Build history of the part. All positions in model axes, mm. Face numbers are marked on the shaded views. A direction names the side the tool comes from. Round coordinates to 2 decimals unless told otherwise and drop trailing zeros. Order: outer loops, then holes, each group sorted by start corner. A loop starts at its lowest first (then second) coordinate and runs counter-clockwise, first axis right, second up. Notation, with made-up numbers: M 30,34 L 35,34 A11 cw 35,51 Z; hole C -30,79.5 d4. An arc over 180 degrees is marked long. Use CSV: the item, a comma, the result in double quotes.
from build123d import *

# Parameters (mm, degrees)
SKETCH_1_W          = 26
SKETCH_1_H          = 25
EXTRUDE_1_DEPTH     = 20
EXTRUDE_3_DEPTH     = 26
SKETCH_4_W          = 26
SKETCH_4_H          = 18
EXTRUDE_4_DEPTH     = 10
SKETCH_5_W          = 22.5
SKETCH_5_H          = 12.5
CUT_EXTRUDE_1_DEPTH = 23.05
CUT_EXTRUDE_5_DEPTH = 3.55
SKETCH_9_W          = 7
SKETCH_9_H          = 8
CUT_EXTRUDE_6_DEPTH = 2
SKETCH_10_W         = 2
SKETCH_10_H         = 8
CUT_EXTRUDE_7_DEPTH = 2
EXTRUDE_5_DEPTH     = 26
FILLET_1_R          = 2


with BuildPart() as part:
    # Эскиз1 → Бобышка-Вытянуть1 (new body)
    with BuildSketch(Plane.XY):
        Rectangle(SKETCH_1_W, SKETCH_1_H)
    extrude(amount=EXTRUDE_1_DEPTH)

    # Эскиз3 → Бобышка-Вытянуть3 (add, through all)
    with BuildSketch(Plane(origin=(13, 0, 0), x_dir=(0, 0, -1), z_dir=(1, 0, 0))):
        with BuildLine():
            Line((-20, 12.5), (-21.75, 12.5))
            ThreePointArc((-21.75, 12.5), (-23, 11.25), (-21.75, 10))
            Line((-21.75, 10), (-20, 10))
            Line((-20, 10), (-20, 12.5))
        make_face()
    extrude_3 = extrude(amount=-EXTRUDE_3_DEPTH)

    # Зеркальное отражение1: Бобышка-Вытянуть3 across plane
    add(extrude_3.mirror(Plane.ZX))

    # Эскиз4 → Бобышка-Вытянуть4 (add)
    with BuildSketch(Plane.XY.offset(20)):
        Rectangle(SKETCH_4_W, SKETCH_4_H)
    extrude(amount=EXTRUDE_4_DEPTH)

    # Эскиз5 → Вырез-Вытянуть1 (cut)
    with BuildSketch(Plane.XY.offset(30)):
        Rectangle(SKETCH_5_W, SKETCH_5_H)
    extrude(amount=-CUT_EXTRUDE_1_DEPTH, mode=Mode.SUBTRACT)

    # Эскиз8 → Вырез-Вытянуть5 (cut)
    with BuildSketch(Plane.ZY.offset(13)):
        with BuildLine():
            Line((30, -6.25), (13.2, -6.25))
            ThreePointArc((13.2, -6.25), (6.95, 0), (13.2, 6.25))
            Line((13.2, 6.25), (30, 6.25))
            Line((30, 6.25), (30, -6.25))
        make_face()
    extrude(amount=-CUT_EXTRUDE_5_DEPTH, mode=Mode.SUBTRACT)

    # Эскиз9 → Вырез-Вытянуть6 (cut)
    with BuildSketch(Plane.XY.offset(6.95)):
        with Locations((7.7560221, 0)):
            Rectangle(SKETCH_9_W, SKETCH_9_H)
    extrude(amount=-CUT_EXTRUDE_6_DEPTH, mode=Mode.SUBTRACT)

    # Эскиз10 → Вырез-Вытянуть7 (cut)
    with BuildSketch(Plane.ZY.offset(-11.2560221)):
        with Locations((5.95, 0)):
            Rectangle(SKETCH_10_W, SKETCH_10_H)
    extrude(amount=-CUT_EXTRUDE_7_DEPTH, mode=Mode.SUBTRACT)

    # Эскиз12 → Бобышка-Вытянуть5 (add, through all)
    with BuildSketch(Plane(origin=(13, 0, 0), x_dir=(0, 0, -1), z_dir=(1, 0, 0))):
        Polygon((-30, 9), (-32.5, 9), (-32.5, 6.25), (-31.2, 6.25), (-31.2, 7.5), (-30, 7.5), align=None)
    extrude_5 = extrude(amount=-EXTRUDE_5_DEPTH)

    # Зеркальное отражение2: Бобышка-Вытянуть5 across plane
    add(extrude_5.mirror(Plane.ZX))

    # Скругление1
    fillet_1_edges = [part.edges().sort_by_distance(p)[0] for p in [
        (0, 12.5, 0),
        (0, -12.5, 0),
    ]]
    fillet(fillet_1_edges, radius=FILLET_1_R)


solid = part.part
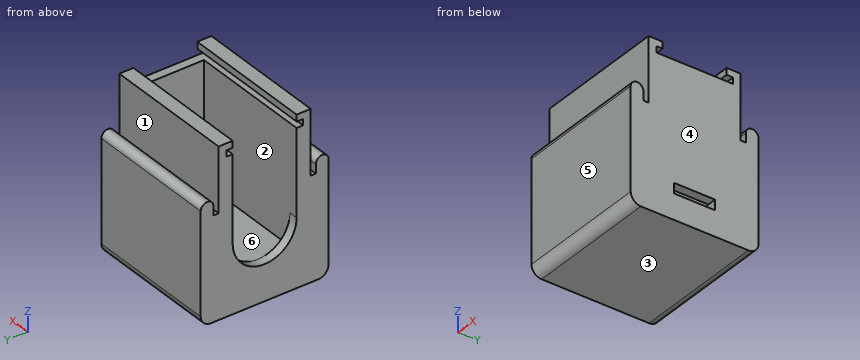
(1) Drop flat-ended pins along their axis: pin 1 (6 mm diameter, centred on x = -1.5, z = 25, fed in from +Y); pin 2 (2 mm diameter, centred on x = -2, y = -1.5, fed in from +Z); pin 3 (6 mm diameter, centred on y = 0, z = 15.5, fed in from -X). Give the stop position or say it passes through.
Answer block:
pin 1,"stops at y = 12.47"
pin 2,"stops at z = 6.95"
pin 3,"stops at x = 11.25"
(2) Two-plate mould, pull along Y, no slides. Class the marked faces 4, 5 and 6: released by +Y, released by -Y, zero draft, split by the parting line, or undercut.
Answer block:
face 4,"zero draft"
face 5,"released by -Y"
face 6,"undercut"
(3) Wall check: line 1 (Y direction, x = 3, z = 21); line 2 (Y direction, x = -3.75, z = 27); line 3 (Y direction, x = 1.5, z = 11). Give the ranges that are in metal, low to high. Write a range as from..to.
Answer block:
line 1,"y = -12.5..-10, -9..-6.25, 6.25..9, 10..12.5"
line 2,"y = -9..-6.25, 6.25..9"
line 3,"y = -12.5..-6.25, 6.25..12.5"
(4) Cut at D-D, the plane y = 1.5. Give the cut face in (x, z).
Answer block:
outline,"M -13,0 L 13,0 L 13,4.95 L 4.26,4.95 L 4.26,6.95 L -11.25,6.95 L -11.25,7.13 L -13,7.13 Z; M 11.25,6.95 L 13,6.95 L 13,30 L 11.25,30 Z"
(5) Cut at B-B, the plane z = 29.5. Give the cut face in (x, y).
Answer block:
outline,"M -13,-9 L 13,-9 L 13,9 L -13,9 L -13,6.25 L 11.25,6.25 L 11.25,-6.25 L -13,-6.25 Z"
(6) Tool access for the marked faces 1, 2 and 3: list every direction of +Z, -Z, +X, -X, +Y, -Y with a clear straight run to the whole face (end or side of a thin tool).
Answer block:
face 1,"+Z, +X, -X"
face 2,"+Z"
face 3,"-Z, +X, -X, +Y, -Y"
(7) Cut at A-A, the plane y = -2.5. Give the cut face in (x, z).
Answer block:
outline,"M -13,0 L 13,0 L 13,4.95 L 4.26,4.95 L 4.26,6.95 L -11.25,6.95 L -11.25,7.47 L -13,7.47 Z; M 11.25,6.95 L 13,6.95 L 13,30 L 11.25,30 Z"
